Input: part model. Units: mm. Frame: model coordinates. Face numbers are marked on the shaded views. A direction names the side the tool comes from. Round coordinates to 2 decimals unless told otherwise and drop trailing zeros. Loops run counter-clockwise (first coordinate to the right, second up) from the corner with the lowest first, then second, coordinate; pieces in that order, holes last. Notation, with made-up numbers: M 14,-4.75 L 51,-4.75 A18 ccw 51,15.25 Z; hole C 83,15 d10. An arc over 180 degrees is marked long. Use one line per item in the form item = value. Start each with the question number.
Q1. First-contact query: P1, Ø8, axis at x = 79, y = 89, coming from the +Z side; P2, Ø6, axis at x = 30.5, y = 98, coming from the -Z side; P3, Ø10, axis at y = 95, z = 66, coming from the +X side. Flat tips, straight axial feed; report the tip coordinate or a pass-through.
Q2. Section query A-A, the plane z = 32. Output: boundary loops of the cut face in (x, y), and give its area (3 significant figures).
Q3. Section query B-B, the plane x = 7.5. Output: boundary loops of the cut face in (y, z).
Q4. Access query for the marked faces 1, 2 and 3. Directions: +Z, -Z, +X, -X, +Y, -Y. A direction counts if a zero-diameter tool reaches every point of the face in a straight line with its end or side. Return the directions, or none.
Q5. Mould query, pull axis Y, two halves, no side actions, for the marked faces 4, 5, 6 and 7. Classes: pulls with the +Y half, pulls with the -Y half, needs draft (parallel to the pull), parting line crosses it, or undercut.
Q6. Ray query, line 1 along Y through (x, z) = (60, 63); line 2 along Y through (x, z) = (66, 17); line 3 along Y through (x, z) = (111, 24). Return the intervals inside material, ascending.
Q7. Section query C-C, the plane z = 64.5. Output: boundary loops of the cut face in (x, y).
```python
from build123d import *

# Parameters (mm, degrees)
SKETCH2_W           = 120
SKETCH2_H           = 120
BOSS_EXTRUDE1_DEPTH = 50
SKETCH4_R           = 35
BOSS_EXTRUDE2_DEPTH = 25
SKETCH6_R           = 25
CUT_EXTRUDE1_DEPTH  = 186.539753153
FILLET1_R           = 5
FILLET2_R           = 1.5
SHELL1_T            = -2


with BuildPart() as part:
    # Sketch2 → Boss-Extrude1 (new body)
    with BuildSketch(Plane.XY):
        with Locations((60, 60)):
            Rectangle(SKETCH2_W, SKETCH2_H)
    extrude(amount=BOSS_EXTRUDE1_DEPTH)

    # Sketch4 → Boss-Extrude2 (add)
    with BuildSketch(Plane.XY.offset(50)):
        with Locations(Location((60, 60, 0), (0, 0, 180))):
            Circle(SKETCH4_R)
    extrude(amount=BOSS_EXTRUDE2_DEPTH)

    # Sketch6 → Cut-Extrude1 (cut, through all)
    with BuildSketch(Plane.XY.offset(75)):
        with Locations((60, 60)):
            Circle(SKETCH6_R)
    extrude(amount=-CUT_EXTRUDE1_DEPTH, mode=Mode.SUBTRACT)

    # Fillet1
    fillet1_edges = [part.edges().sort_by_distance(p)[0] for p in [
        (120, 60, 50),
        (60, 120, 50),
        (95, 60, 50),
        (0, 60, 50),
        (60, 0, 50),
        (0, 120, 25),
        (120, 120, 25),
        (120, 0, 25),
        (0, 0, 25),
    ]]
    fillet(fillet1_edges, radius=FILLET1_R)

    # Fillet2
    fillet2_edges = [part.edges().sort_by_distance(p)[0] for p in [
        (95, 60, 75),
        (35, 60, 75),
    ]]
    fillet(fillet2_edges, radius=FILLET2_R)

    # Shell1
    shell1_openings = [part.faces().sort_by_distance(p)[0] for p in [
        (60, 1.697056275, 0),
    ]]
    offset(amount=SHELL1_T, openings=shell1_openings, kind=Kind.INTERSECTION)


solid = part.part
```
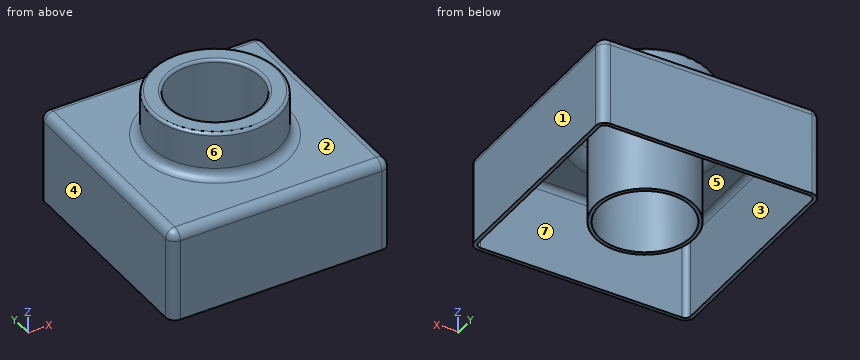
Results found:
q1.P1 = 75
q1.P2 = 48
q1.P3 = 78.03
q2.outline = M 0,5 A5 ccw 5,0 L 115,0 A5 ccw 120,5 L 120,115 A5 ccw 115,120 L 5,120 A5 ccw 0,115 Z; C 60,60 d54; hole M 2,5 A3 ccw 5,2 L 115,2 A3 ccw 118,5 L 118,115 A3 ccw 115,118 L 5,118 A3 ccw 2,115 Z; hole C 60,60 d50
q2.area = 1,260 mm²
q3.outline = M 0,0 L 2,0 L 2,45 A3 cw 5,48 L 115,48 A3 cw 118,45 L 118,0 L 120,0 L 120,45 A5 ccw 115,50 L 5,50 A5 ccw 0,45 Z
q4.face_1 = +Z, -Z, +X, +Y, -Y
q4.face_2 = +Z
q4.face_3 = -Z
q5.face_4 = needs draft
q5.face_5 = undercut
q5.face_6 = parting line crosses it
q5.face_7 = undercut
q6.line_1 = 25 to 27, 33 to 35, 85 to 87, 93 to 95
q6.line_2 = 0 to 2, 33.68 to 35.73, 84.27 to 86.32, 118 to 120
q6.line_3 = 0 to 2, 118 to 120
q7.outline = C 60,60 d70; C 60,60 d54; hole C 60,60 d66; hole C 60,60 d50
